Here's how the part is built. I have some questions about the finished solid (model axes, mm). Round coordinates to 2 decimals unless told otherwise and drop trailing zeros. Write each loop counter-clockwise with the first axis right and the second up, starting at its lowest first coordinate (ties: lowest second). Pieces come first, ordered by that corner, then holes. Notation, with made-up numbers: (9.5, -38.75) -> (31.5, -38.75) arc R23 ccw to (31.5, -23.75) -> close; hole circle Ø5 at (38.5, 2). An arc over 180 degrees is marked (long way). Answer as CSV lines item,"result".
```python
from build123d import *

# Parameters (mm, degrees)
SKETCH1_R           = 32.5
SKETCH1_R_2         = 3.1
SKETCH1_R_3         = 2.25
BOSS_EXTRUDE1_DEPTH = 5
CHAMFER1_SIZE       = 3.3
CHAMFER2_SIZE       = 1


with BuildPart() as part:
    # Sketch1 → Boss-Extrude1 (new body)
    with BuildSketch(Plane(origin=(0, 0, 0), x_dir=(1, 0, 0), z_dir=(0, 1, 0))):
        with Locations(Location((0, 0, 0), (0, 0, 270))):
            Circle(SKETCH1_R)
        with Locations(Location((0, 25, 0), (0, 0, 270))):
            Circle(SKETCH1_R_2, mode=Mode.SUBTRACT)
        with Locations(Location((25, 0, 0), (0, 0, 270))):
            Circle(SKETCH1_R_2, mode=Mode.SUBTRACT)
        with Locations(Location((0, -25, 0), (0, 0, 270))):
            Circle(SKETCH1_R_2, mode=Mode.SUBTRACT)
        with Locations(Location((-25, 0, 0), (0, 0, 270))):
            Circle(SKETCH1_R_2, mode=Mode.SUBTRACT)
        with Locations(Location((-17.67766953, 17.67766953, 0), (0, 0, 270))):
            Circle(SKETCH1_R_3, mode=Mode.SUBTRACT)
        with Locations(Location((17.67766953, -17.67766953, 0), (0, 0, 270))):
            Circle(SKETCH1_R_3, mode=Mode.SUBTRACT)
    extrude(amount=BOSS_EXTRUDE1_DEPTH)

    # Chamfer1
    chamfer1_edges = [part.edges().sort_by_distance(p)[0] for p in [
        (25, 0, -3.1),
        (0, 0, 21.9),
        (-25, 0, -3.1),
        (0, 0, -28.1),
    ]]
    chamfer(chamfer1_edges, length=CHAMFER1_SIZE)

    # Chamfer2
    chamfer2_edges = [part.edges().sort_by_distance(p)[0] for p in [
        (0, 0, -32.5),
        (0, 5, -32.5),
    ]]
    chamfer(chamfer2_edges, length=CHAMFER2_SIZE)


solid = part.part
```
1. If I drill on line 1 (X direction, y = 1.7, z = 2); line 2 (X direction, y = 3.5, z = -1.5); line 3 (Z direction, x = 3, y = 2.75), over which ranges is the centre line in solid material (lowest first)?
Numbers:
line 1,"x = -32.44 to -29.25, -20.75 to 20.75, 29.25 to 32.44"
line 2,"x = -32.47 to -27.71, -22.29 to 22.29, 27.71 to 32.47"
line 3,"z = -32.36 to -27.08, -22.92 to 22.92, 27.08 to 32.36"
2. Suppose I cut it at B-B on x = 0. Please give me the cut outline in (y, z), and give its area (3 significant figures).
Numbers:
outline,"(0, -31.5) -> (1, -32.5) -> (4, -32.5) -> (5, -31.5) -> (5, -28.1) -> (3.3, -28.1) -> (0, -31.4) -> close; (0, -18.6) -> (3.3, -21.9) -> (5, -21.9) -> (5, 21.9) -> (3.3, 21.9) -> (0, 18.6) -> close; (0, 31.4) -> (3.3, 28.1) -> (5, 28.1) -> (5, 31.5) -> (4, 32.5) -> (1, 32.5) -> (0, 31.5) -> close"
area,"239 mm^2"
3. For pin 1 Ø2.5 at (x, z) = (-17.68, -17.68) entering from -Y; pin 2 Ø7 at (x, z) = (0, 25) entering from -Y; pin 3 Ø1 at (x, z) = (23.5, -3) entering from -Y; pin 4 Ø1 at (x, y) = (5.5, 3.5) entering from +Z, each with a flat end and sliding along its axis, tell me the tip position at first contact or that it passes through.
Numbers:
pin 1,"passes through"
pin 2,"stops at y = 2.9"
pin 3,"stops at y = 2.55"
pin 4,"stops at z = 32.11"
4. Suppose I cut it at A-A on z = 0. Please give me the cut outline in (x, y), and give its area (3 significant figures).
Numbers:
outline,"(-32.5, 1) -> (-31.5, 0) -> (-31.4, 0) -> (-28.1, 3.3) -> (-28.1, 5) -> (-31.5, 5) -> (-32.5, 4) -> close; (-21.9, 3.3) -> (-18.6, 0) -> (18.6, 0) -> (21.9, 3.3) -> (21.9, 5) -> (-21.9, 5) -> close; (28.1, 3.3) -> (31.4, 0) -> (31.5, 0) -> (32.5, 1) -> (32.5, 4) -> (31.5, 5) -> (28.1, 5) -> close"
area,"239 mm^2"
5. If we mould it in two halves opening along X, with no side actions, what happens to faces 1 (the face through (0, 5, 0)), 2 (the face through (0.993, 3.094, 28.154)), 3 (the face through (9.76, 2.48, 31))? For each: released by +X, released by -X, zero draft, split by the parting line, or undercut.
Numbers:
face 1,"zero draft"
face 2,"undercut"
face 3,"split by the parting line"
